Part model, mm, in its own coordinate system. Give positions to 0.01 mm unless a question says otherwise; leave off trailing zeros. Loops run counter-clockwise (first coordinate to the right, second up) from the corner with the lowest first, then second, coordinate; pieces in that order, holes last. Notation, with made-up numbers: (81.25, 50.25) -> (109.25, 50.25) arc R27 cw to (109.25, 75.25) -> close; hole circle Ø11 at (-6, -15.5). An arc over 180 degrees is marked (long way). One line per question, with ' | ' between items.
```python
from build123d import *

# Parameters (mm, degrees)
BOSS_EXTRUDE1_DEPTH            = 9.525
V_0_377_DIAMETER_SLOT2_DEPTH   = 9.525
CUT_EXTRUDE1_REACH             = 358.93
SKETCH6_W                      = 152.4
SKETCH6_H                      = 622.3
FILLET1_R                      = 12.7
SKETCH7_R                      = 8.382
CUT_EXTRUDE2_DEPTH             = 357.929879318
SKETCH12_W                     = 38.1
SKETCH12_H                     = 107.95
SKETCH12_H_2                   = 82.55
CUT_EXTRUDE3_DEPTH             = 357.929879318
FILLET2_R                      = 6.35
F_5_16_0_3125_DIAMETER_HOLE1_D = 7.9375
SKETCH16_W                     = 158.75
SKETCH16_H                     = 26.277954941
CUT_EXTRUDE4_DEPTH             = 357.929879318
F_5_16_0_3125_DIAMETER_HOLE2_D = 7.9375
FILLET3_R                      = 12.7
CUT_EXTRUDE5_DEPTH             = 1.27


# Read off the part's stored shape, not the designer's step: V (0.377) Diameter Slot2
with BuildPart() as part:
    # Sketch1 → Boss-Extrude1 (new body)
    with BuildSketch(Plane.XY):
        with BuildLine():
            Line((-174.625, 151.522045059), (-174.625, 311.15))
            Line((-174.625, 311.15), (174.625, 311.15))
            Line((174.625, 311.15), (174.625, 151.522045059))
            ThreePointArc((174.625, 151.522045059), (66.675, -31.75), (174.625, -215.022045059))
            Line((174.625, -215.022045059), (174.625, -311.15))
            Line((174.625, -311.15), (-174.625, -311.15))
            Line((-174.625, -311.15), (-174.625, -215.022045059))
            ThreePointArc((-174.625, -215.022045059), (-66.675, -31.75), (-174.625, 151.522045059))
        make_face()
    extrude(amount=BOSS_EXTRUDE1_DEPTH)

    # V (0.377) Diameter Slot2 outline → V (0.377) Diameter Slot2 (cut)
    with BuildSketch(Plane.XY):
        with BuildLine():
            Line((4.7879, -57.8866), (4.7879, -45.2374))
            ThreePointArc((4.7879, -45.2374), (0, -40.4495), (-4.7879, -45.2374))
            Line((-4.7879, -45.2374), (-4.7879, -57.8866))
            ThreePointArc((-4.7879, -57.8866), (0, -62.6745), (4.7879, -57.8866))
        make_face()
        with BuildLine():
            ThreePointArc((4.7879, 94.4626), (0, 99.2505), (-4.7879, 94.4626))
            Line((-4.7879, 94.4626), (-4.7879, 81.8134))
            ThreePointArc((-4.7879, 81.8134), (0, 77.0255), (4.7879, 81.8134))
            Line((4.7879, 81.8134), (4.7879, 94.4626))
        make_face()
        with BuildLine():
            ThreePointArc((4.7879, -184.9374), (0, -180.1495), (-4.7879, -184.9374))
            Line((-4.7879, -184.9374), (-4.7879, -197.5866))
            ThreePointArc((-4.7879, -197.5866), (0, -202.3745), (4.7879, -197.5866))
            Line((4.7879, -197.5866), (4.7879, -184.9374))
        make_face()
    extrude(amount=V_0_377_DIAMETER_SLOT2_DEPTH, mode=Mode.SUBTRACT)

    # Sketch6 → Cut-Extrude1 (cut, up to next)
    with BuildSketch(Plane.XY.offset(9.525), mode=Mode.PRIVATE) as cut_extrude1_sk1:
        with Locations((-98.425, 0)):
            Rectangle(SKETCH6_W, SKETCH6_H)
    cut_extrude1_tool1 = extrude(cut_extrude1_sk1.sketch, amount=-CUT_EXTRUDE1_REACH, mode=Mode.PRIVATE) & part.part
    add(cut_extrude1_tool1.solids().sort_by_distance((-98.425, 0, 9.525))[0], mode=Mode.SUBTRACT)

    # Fillet1
    fillet1_edges = [part.edges().sort_by_distance(p)[0] for p in [
        (174.625, -311.15, 4.7625),
    ]]
    fillet(fillet1_edges, radius=FILLET1_R)

    # Sketch7 → Cut-Extrude2 (cut, through all)
    with BuildSketch(Plane.XY.offset(9.525)):
        with Locations((0, -197.5866)):
            Circle(SKETCH7_R)
        with Locations((0, 81.8134)):
            Circle(SKETCH7_R)
        with Locations((0, -57.8866)):
            Circle(SKETCH7_R)
    extrude(amount=-CUT_EXTRUDE2_DEPTH, mode=Mode.SUBTRACT)

    # Sketch12 → Cut-Extrude3 (cut, through all)
    with BuildSketch(Plane.XY.offset(9.525)):
        with Locations((-3.175, 257.175)):
            Rectangle(SKETCH12_W, SKETCH12_H)
        with Locations((-3.175, -269.875)):
            Rectangle(SKETCH12_W, SKETCH12_H_2)
    extrude(amount=-CUT_EXTRUDE3_DEPTH, mode=Mode.SUBTRACT)

    # Fillet2
    fillet2_edges = [part.edges().sort_by_distance(p)[0] for p in [
        (15.875, 203.2, 4.7625),
        (15.875, -228.6, 4.7625),
    ]]
    fillet(fillet2_edges, radius=FILLET2_R)

    # 5/16 (0.3125) Diameter Hole1 (through all)
    with Locations(Plane.XY.offset(9.525)):
        with Locations((85.7885, 170.688), (85.7885, 265.938)):
            Hole(F_5_16_0_3125_DIAMETER_HOLE1_D / 2)

    # Sketch16 → Cut-Extrude4 (cut, through all)
    with BuildSketch(Plane.XY.offset(9.525)):
        with Locations((95.25, 298.011022529)):
            Rectangle(SKETCH16_W, SKETCH16_H)
    extrude(amount=-CUT_EXTRUDE4_DEPTH, mode=Mode.SUBTRACT)

    # 5/16 (0.3125) Diameter Hole2 (through all)
    with Locations(Plane.XY.offset(9.525)):
        with Locations((85.7885, -234.95), (85.7885, -292.1)):
            Hole(F_5_16_0_3125_DIAMETER_HOLE2_D / 2)

    # Fillet3
    fillet3_edges = [part.edges().sort_by_distance(p)[0] for p in [
        (174.625, 284.872045059, 4.7625),
    ]]
    fillet(fillet3_edges, radius=FILLET3_R)

    # Sketch22 → Cut-Extrude5 (cut)
    with BuildSketch(Plane(origin=(0, 0, 0), x_dir=(-1, 0, 0), z_dir=(0, 0, -1))):
        with BuildLine():
            Line((4.803205128, 190.5), (7.344731571, 190.5))
            add(Edge.make_bspline(
                [(7.344731571, 190.5), (7.514335094, 190.499435445), (7.839992647, 190.498351437), (8.306529942, 190.492307098), (8.730445408, 190.474983007), (9.111517396, 190.460074718), (9.449738916, 190.432889674), (9.746147085, 190.406906754), (9.99937673, 190.372893757), (10.152668819, 190.341305508), (10.222075321, 190.327003205)],
                knots=[0, 0, 0, 0, 1.410062039, 2.707475311, 3.878576406, 4.937260626, 5.877586885, 6.699081471, 7.410979367, 8, 8, 8, 8], degree=3))
            add(Edge.make_bspline(
                [(10.222075321, 190.327003205), (10.314990785, 190.304046085), (10.498839576, 190.258621583), (10.763544101, 190.162611031), (11.015781791, 190.051505536), (11.254504868, 189.921008608), (11.478517596, 189.77015155), (11.690129752, 189.601538649), (11.890301576, 189.416092502), (12.070937777, 189.209137506), (12.241259479, 188.992016457), (12.384909638, 188.757234253), (12.508740007, 188.511719568), (12.607330169, 188.252975509), (12.686715958, 187.983511365), (12.74269117, 187.700886303), (12.776259765, 187.406387908), (12.779677355, 187.205517781), (12.781410256, 187.103665865)],
                knots=[0, 0, 0, 0, 1.027469482, 2.033020251, 3.019912614, 3.986113645, 4.951240523, 5.91722682, 6.890402269, 7.87763091, 8.8651537, 9.85103654, 10.82876324, 11.815024772, 12.821070561, 13.842952187, 14.906261191, 16, 16, 16, 16], degree=3))
            add(Edge.make_bspline(
                [(12.781410256, 187.103665865), (12.776079892, 186.934447057), (12.76567897, 186.604257334), (12.668705022, 186.125064993), (12.509858794, 185.678063765), (12.290971431, 185.263816479), (12.012226476, 184.890397852), (11.677219377, 184.562409628), (11.285763244, 184.287944802), (10.921348297, 184.097616054), (10.599442487, 183.975721785), (10.334435895, 183.889955569), (10.045358576, 183.823690724), (9.734980248, 183.764326817), (9.40200927, 183.719507811), (9.047243698, 183.686681597), (8.670430519, 183.666165478), (8.41157161, 183.663110203), (8.278405449, 183.661538462)],
                knots=[0, 0, 0, 0, 1.260483769, 2.459530307, 3.627416485, 4.787058657, 5.939039949, 7.08810263, 8.267026773, 9.491475466, 10.141966685, 10.831826277, 11.566392101, 12.351337768, 13.187381173, 14.07005841, 15.007169909, 16, 16, 16, 16], degree=3))
            Line((8.278405449, 183.661538462), (12.944230769, 177.8))
            Line((12.944230769, 177.8), (11.534815705, 177.8))
            Line((11.534815705, 177.8), (6.868990385, 183.661538462))
            Line((6.868990385, 183.661538462), (5.942948718, 183.661538462))
            Line((5.942948718, 183.661538462), (5.942948718, 177.8))
            Line((5.942948718, 177.8), (4.803205128, 177.8))
            Line((4.803205128, 177.8), (4.803205128, 190.5))
        make_face()
        with BuildLine():
            Line((5.942948718, 189.197435897), (5.942948718, 184.964102564))
            Line((5.942948718, 184.964102564), (8.268229167, 184.946294071))
            add(Edge.make_bspline(
                [(8.268229167, 184.946294071), (8.376796165, 184.94624604), (8.587229929, 184.946152944), (8.891669485, 184.960644647), (9.17513389, 184.977130401), (9.436538905, 185.002346598), (9.676001307, 185.034844344), (9.893401406, 185.075495173), (10.08909408, 185.122855514), (10.31732592, 185.196158556), (10.572184191, 185.31229468), (10.849158345, 185.481260918), (11.085023971, 185.69378315), (11.284297357, 185.936801119), (11.444424151, 186.203995508), (11.557316462, 186.492163476), (11.628953324, 186.794030132), (11.637402618, 187.00150498), (11.641666667, 187.106209936)],
                knots=[0, 0, 0, 0, 1.146690395, 2.22261258, 3.21895312, 4.145990853, 4.996080663, 5.770904154, 6.481378293, 7.121626537, 8.300444488, 9.431385265, 10.535395872, 11.636531494, 12.74115979, 13.810798291, 14.895190096, 16, 16, 16, 16], degree=3))
            add(Edge.make_bspline(
                [(11.641666667, 187.106209936), (11.637304684, 187.208341789), (11.628660827, 187.410729855), (11.558089581, 187.707024158), (11.438748112, 187.986667092), (11.277921706, 188.24852108), (11.081981915, 188.486213322), (10.852228709, 188.68958442), (10.594944144, 188.857403906), (10.354474367, 188.964644087), (10.139538796, 189.030393268), (9.952922601, 189.076661777), (9.742060953, 189.113834564), (9.505930003, 189.143618099), (9.2455378, 189.169217469), (8.959567723, 189.186459637), (8.649917121, 189.196669944), (8.435298256, 189.197174638), (8.324198718, 189.197435897)],
                knots=[0, 0, 0, 0, 1.101028733, 2.181837193, 3.264309656, 4.369019818, 5.486613113, 6.575447106, 7.666700264, 8.788928104, 9.402425223, 10.0903467, 10.862060571, 11.710948788, 12.657782767, 13.684531032, 14.801375019, 16, 16, 16, 16], degree=3))
            Line((8.324198718, 189.197435897), (5.942948718, 189.197435897))
        make_face(mode=Mode.SUBTRACT)
    extrude(amount=-CUT_EXTRUDE5_DEPTH, mode=Mode.SUBTRACT)


solid = part.part
```
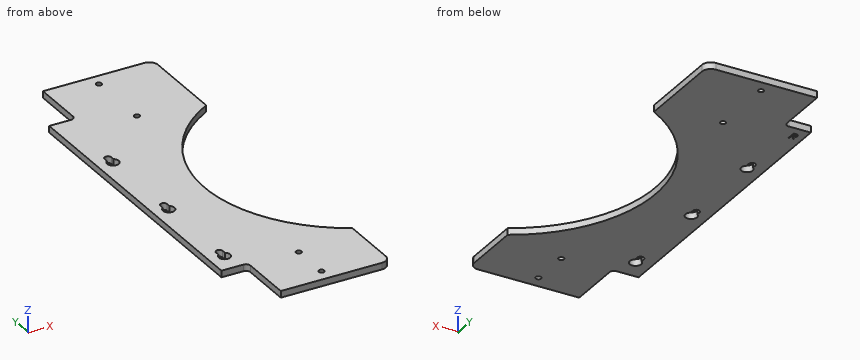
1) Saw through at A-A (z = 7.25). State how many separate pieces and enclosed holes the cut face has, and give its area (3 significant figures).
Found:
separate pieces: 1 | enclosed holes: 7 | area: 81,800 mm2
2) Saw through at B-B (y = -151). Give the cut face in (x, z) (3 decimals), and give its area (3 significant figures).
Found:
outline: (-22.225, 0) -> (103.915, 0) -> (103.915, 9.525) -> (-22.225, 9.525) -> close | area: 1,200 mm2
3) Pin check, flat tips, straight feed: P1, Ø3, axis at y = -198, z = 2, coming from the +X side; P2, Ø5, axis at x = 4, y = -121, coming from the -Z side; P3, Ø5, axis at y = 247.5, z = 7, coming from the -X side (3 decimals); P4, Ø1.7, axis at y = -187.5, z = 2.5, coming from the +X side. Stop position of each tip, or through.
Found:
P1: x = 150.64 | P2: z = 0 | P3: x = 15.875 | P4: x = 136.99
4) Drill centre lines: line 1 (Y direction, x = 0, z = 5.5); line 2 (Y direction, x = 6, z = 4); line 3 (Y direction, x = 90, z = 6.5). Where is each one in solid material? Low to high.
Found:
line 1: -228.6 to -205.97, -180.15 to -66.27, -40.45 to 73.43, 99.25 to 203.2 | line 2: -228.6 to -203.44, -191.73 to -63.74, -52.03 to 75.96, 87.67 to 203.2 | line 3: -311.15 to -127.83, 64.33 to 284.87
